from build123d import *

# Parameters (mm, degrees)
BASPROSKE_W         = 10
BASPROSKE_H         = 19.25
TOOTHCUT_DEPTH      = 30.002155092
TEETHCUTS_COUNT     = 20
TEETHCUTS_ANGLE     = 342
BORSKE_R            = 0.4
BORE_DEPTH          = 50.0000508
SKETCH1_R           = 2.5
CUT_EXTRUDE1_DEPTH  = 29.779222719
CUT_EXTRUDE_1_DEPTH = 5.5
SKETCH_4_R          = 25
CUT_EXTRUDE_2_DEPTH = 4.5


with BuildPart() as part:
    # BasProSke → Base-Revolve (revolve)
    with BuildSketch(Plane(origin=(0, 0, 0), x_dir=(1, 0, 0), z_dir=(0, 1, 0)), mode=Mode.PRIVATE) as base_revolve_sk:
        with Locations((5, 9.625)):
            Rectangle(BASPROSKE_W, BASPROSKE_H)
    revolve(base_revolve_sk.sketch.rotate(Axis((-10, 0, 0), (1, 0, 0)), 180), axis=Axis((-10, 0, 0), (1, 0, 0)))

    # TooCutSke → ToothCut (cut, through all)
    with BuildSketch(Plane(origin=(0, 0, 0), x_dir=(0, 0, -1), z_dir=(1, 0, 0))):
        with BuildLine():
            ThreePointArc((0.85426341, 15.287650777), (0, 15.3115), (-0.85426341, 15.287650777))
            ThreePointArc((-0.85426341, 15.287650777), (-1.414533498, 17.326428412), (-2.557997552, 19.104912815))
            ThreePointArc((-2.557997552, 19.104912815), (0, 19.2754), (2.557997552, 19.104912815))
            ThreePointArc((2.557997552, 19.104912815), (1.414533498, 17.326428412), (0.85426341, 15.287650777))
        make_face()
    toothcut = extrude(amount=TOOTHCUT_DEPTH, mode=Mode.SUBTRACT)

    # TeethCuts: ToothCut ×20 about axis
    teethcuts_axis = Axis((-10, 0, 0), (1, 0, 0))
    for i in range(1, TEETHCUTS_COUNT):
        add(toothcut.rotate(teethcuts_axis, i * TEETHCUTS_ANGLE / (TEETHCUTS_COUNT - 1)), mode=Mode.SUBTRACT)

    # BorSke → Bore (cut, symmetric)
    with BuildSketch(Plane(origin=(0, 0, 0), x_dir=(0, 0, -1), z_dir=(1, 0, 0))):
        with Locations(Location((0, 0, 0), (0, 0, 180))):
            Circle(BORSKE_R)
    extrude(amount=BORE_DEPTH, both=True, mode=Mode.SUBTRACT)

    # Sketch1 → Cut-Extrude1 (cut, through all)
    with BuildSketch(Plane(origin=(10, 0, 0), x_dir=(0, 0, -1), z_dir=(1, 0, 0))):
        Circle(SKETCH1_R)
    extrude(amount=-CUT_EXTRUDE1_DEPTH, mode=Mode.SUBTRACT)

    # 草图2 → 切除-拉伸1 (cut)
    with BuildSketch(Plane(origin=(10, 0, 0), x_dir=(0, 0, -1), z_dir=(1, 0, 0))):
        with BuildLine():
            ThreePointArc((0.185768463, 3.495066534), (-2.408299232, 2.539703685), (-3.5, 0))
            Line((-3.5, 0), (9.5, 0))
            Line((9.5, 0), (9.5, 3))
            Line((9.5, 3), (0.185768463, 3.495066534))
        make_face()
        with BuildLine():
            Line((9.5, 0), (-3.5, 0))
            ThreePointArc((-3.5, 0), (-2.408299232, -2.539703685), (0.185768463, -3.495066534))
            Line((0.185768463, -3.495066534), (9.5, -3))
            Line((9.5, -3), (9.5, 0))
        make_face()
    extrude(amount=-CUT_EXTRUDE_1_DEPTH, mode=Mode.SUBTRACT)

    # 草图4 → 切除-拉伸2 (cut)
    with BuildSketch(Plane.ZY):
        Circle(SKETCH_4_R)
    extrude(amount=-CUT_EXTRUDE_2_DEPTH, mode=Mode.SUBTRACT)


solid = part.part
Read the model definition and answer for the solid it produces. Units are mm, in the model's axes. A direction names the side the tool comes from. Round coordinates to 2 decimals unless told otherwise and drop trailing zeros. Loops run counter-clockwise (first coordinate to the right, second up) from the corner with the lowest first, then second, coordinate; pieces in that order, holes last.
Q1. Section C-C on y = 4.5 is taken. Write down the section's boundary in (x, z), and give its area (3 significant figures).
Q2. Section B-B on z = -7.5 is taken. Write down the section's boundary in (x, y), and give its area (3 significant figures).
Q3. Consider probe 1 along Y at (x, z) = (6.2, 15); probe 2 along Z at (x, y) = (6.3, -8.5); probe 3 along Z at (x, y) = (8.2, 13.5). Determine where each line is inside the solid, lowest interval first.
Q4. Section A-A on y = -2 is taken. Write down the section's boundary in (x, z), and give its area (3 significant figures).
Q5. Which of the six approach directions +Z, -Z, +X, -X, +Y, -Y give full straight-line access (tool end or side, diameter ignored) to faces 5 (the face through (7.212, 13.193, -11.341)), 6 (the face through (10, 4, 0)), 7 (the face through (7.212, 11.29, -13.163)), 8 (the face through (7.21, 1.42, 17.34)), 9 (the face through (7.21, -14.81, 9.03))?
Q6. Each of these flat-tipped pins is pushed along its axis until it touches: pin 1 (3 mm diameter, centred on x = 5.5, y = 7, fed in from -Z); pin 2 (3 mm diameter, centred on x = 8.5, z = -9.5, fed in from -Y). Where does it stop, or does it pass through?
Q7. Determine the mould class of faces 1 (the face through (7.21, -6.71, -16.05)), 2 (the face through (7.212, -8.99, 12.394)), 3 (the face through (7.212, -13.193, 11.341)), 4 (the face through (7.288, -8.733, 17.155)) for opening direction Z: released by +Z, released by -Z, zero draft, split by the parting line, or undercut.
Output:
1. outline: (4.5, -14.64) - (10, -14.64) - (10, 14.64) - (4.5, 14.64) - close
1. area: 161 mm2
2. outline: (4.5, -16.8) - (10, -16.8) - (10, -3.11) - (4.5, -3.11) - close; (4.5, 3.11) - (10, 3.11) - (10, 16.8) - (4.5, 16.8) - close
2. area: 151 mm2
3. probe 1: y = -9.07 to -5.92, -3.95 to 3.95, 5.92 to 9.07
3. probe 2: z = -17.27 to -13.26, -12.74 to 12.74, 13.26 to 17.27
3. probe 3: z = -13.72 to -11.94, -8.61 to 8.61, 11.94 to 13.72
4. outline: (4.5, -18.38) - (10, -18.38) - (10, -9.5) - (4.5, -9.5) - close; (4.5, 2.87) - (10, 2.87) - (10, 18.38) - (4.5, 18.38) - close
4. area: 134 mm2
5. face 5: +X, -X, +Y
5. face 6: +Z, -Z, +X, +Y, -Y
5. face 7: -Z, +X, -X
5. face 8: +Z, +X, -X
5. face 9: +X, -X
6. pin 1: stops at z = -17.36
6. pin 2: stops at y = -17.36
7. face 1: released by -Z
7. face 2: undercut
7. face 3: undercut
7. face 4: released by +Z
